```python
from build123d import *

# Parameters (mm, degrees)
F1_DEPTH = 8.382
F2_T     = 5.842
F3_W     = 7.7823624015
F3_H     = 6.8200882353
F3_W_2   = 7.1338275447
F3_H_2   = 5.8367699385
F3_W_3   = 11.938
F3_H_3   = 9.4247385517
F4_DEPTH = 5.842


with BuildPart() as f1:
    # F0 (on Front) → F1 (new body)
    with BuildSketch(Plane.XZ):
        with BuildLine():
            Line((-45.2634918147, -64.6201544654), (14.1725081853, -64.6201544654))
            ThreePointArc((14.1725081853, -64.6201544654), (18.6626362458, -62.760282526), (20.5225081853, -58.2701544654))
            Line((20.5225081853, -58.2701544654), (20.5225081853, 71.2698455346))
            ThreePointArc((20.5225081853, 71.2698455346), (18.6626362458, 75.7599735951), (14.1725081853, 77.6198455346))
            Line((14.1725081853, 77.6198455346), (-45.2634918147, 77.6198455346))
            ThreePointArc((-45.2634918147, 77.6198455346), (-49.7536198753, 75.7599735951), (-51.6134918147, 71.2698455346))
            Line((-51.6134918147, 71.2698455346), (-51.6134918147, -58.2701544654))
            ThreePointArc((-51.6134918147, -58.2701544654), (-49.7536198753, -62.760282526), (-45.2634918147, -64.6201544654))
        make_face()
    extrude(amount=F1_DEPTH)

    # F2
    f2_openings = [f1.faces().sort_by_distance(p)[0] for p in [
        (-15.545492, -8.382, 6.499846),
    ]]
    offset(amount=F2_T, openings=f2_openings, kind=Kind.INTERSECTION)

    # F3 (on face) → F4 (cut)
    with BuildSketch(Plane(origin=(0, 5.842, 0), x_dir=(-1, 0, 0), z_dir=(0, 1, 0))):
        with Locations((40.2088426054, 66.2087770264)):
            Rectangle(F3_W, F3_H)
        with Locations((3.5669137724, 66.7004361749)):
            Rectangle(F3_W_2, F3_H_2)
        with Locations((21.0826918147, 67.5111021847)):
            Rectangle(F3_W_3, F3_H_3)
    extrude(amount=-F4_DEPTH, mode=Mode.SUBTRACT)


solid = f1.part
```
Can you work these out from the model? Positions are in its coordinate system, mm. A direction names the side the tool comes from. Coordinates: 2 decimals unless noted, no trailing zeros. Write each loop counter-clockwise with the first axis right and the second up, starting at its lowest first coordinate (ties: lowest second). Pieces come first, ordered by that corner, then holes. Notation, with made-up numbers: (55, 76) - (70, 76) arc R28 cw to (70, 108) - close; hole circle Ø1 at (38, -15). An arc over 180 degrees is marked (long way). Return JSON: item names as keys, results as strings.
Q1. On a 3-axis mill with a long thin cutter (end or side, diameter ignored), from which of +Z, -Z, +X, -X, +Y, -Y can I reach the whole of each face in a straight line? I mean faces 1 (the cylindrical face through (-53.979, -1.17, -66.796)), 2 (the cylindrical face through (-49.704, -4.132, 75.809)), 3 (the flat face through (-15.114, 3, 67)). Say none if no direction works.
Computed values:
{"face 1": "-Z, -X, +Y, -Y", "face 2": "-Y", "face 3": "+Y, -Y"}
Q2. If we section it at C-C (x = 10): Please give me the cut outline in (y, z), then the cut area to 3 significant figures.
Computed values:
{"outline": "(-8.38, -70.46) - (5.84, -70.46) - (5.84, 83.46) - (-8.38, 83.46) - (-8.38, 77.62) - (0, 77.62) - (0, -64.62) - (-8.38, -64.62) - close", "area": "997 mm2"}
Q3. If we section it at B-B (y = 4.25): Please give me the cut outline in (x, z).
Computed values:
{"outline": "(-57.46, -58.27) arc R12.19 ccw to (-45.26, -70.46) - (14.17, -70.46) arc R12.19 ccw to (26.36, -58.27) - (26.36, 71.27) arc R12.19 ccw to (14.17, 83.46) - (-45.26, 83.46) arc R12.19 ccw to (-57.46, 71.27) - close; hole (-44.1, 62.8) - (-36.32, 62.8) - (-36.32, 69.62) - (-44.1, 69.62) - close; hole (-27.05, 62.8) - (-15.11, 62.8) - (-15.11, 72.22) - (-27.05, 72.22) - close; hole (-7.13, 63.78) - (0, 63.78) - (0, 69.62) - (-7.13, 69.62) - close"}
Q4. Thinking about a two-plate mould opening in Z: for faces 4 (the flat face through (-36.318, 3, 66)), 5 (the cylindrical face through (22.888, -1.17, 79.796)), 6 (the flat face through (-57.455, -1, 7)), which applies, +Z half, -Z half, draft (parallel to the pull), parting line (faces both ways), or undercut?
Computed values:
{"face 4": "undercut", "face 5": "+Z half", "face 6": "draft"}
Q5. If we section it at A-A (x = -5): Please give me the cut outline in (y, z), then the cut area to 3 significant figures.
Computed values:
{"outline": "(-8.38, -70.46) - (5.84, -70.46) - (5.84, 63.78) - (0, 63.78) - (0, -64.62) - (-8.38, -64.62) - close; (-8.38, 77.62) - (0, 77.62) - (0, 69.62) - (5.84, 69.62) - (5.84, 83.46) - (-8.38, 83.46) - close", "area": "963 mm2"}
Q6. If we section it at D-D (y = -2.75): Please give me the cut outline in (x, z), then the cut area to 3 significant figures.
Computed values:
{"outline": "(-57.46, -58.27) arc R12.19 ccw to (-45.26, -70.46) - (14.17, -70.46) arc R12.19 ccw to (26.36, -58.27) - (26.36, 71.27) arc R12.19 ccw to (14.17, 83.46) - (-45.26, 83.46) arc R12.19 ccw to (-57.46, 71.27) - close; hole (-51.61, -58.27) arc R6.35 ccw to (-45.26, -64.62) - (14.17, -64.62) arc R6.35 ccw to (20.52, -58.27) - (20.52, 71.27) arc R6.35 ccw to (14.17, 77.62) - (-45.26, 77.62) arc R6.35 ccw to (-51.61, 71.27) - close", "area": "2,550 mm2"}
Q7. I'm going to push a flat-ended pin straight in: pin 1 Ø21.5 at (x, z) = (-16.5, 22) entering from -Y. Where does the tip first touch, or does it pass through?
Computed values:
{"pin 1": "stops at y = 0"}
Q8. Please list where these lines run through material, in increasing order: L1, parallel to X at y = -4, z = 55.5; L2, parallel to Z at x = 12, y = -6; L3, parallel to Z at x = -2, y = 3.75. Write a range as from..to.
Computed values:
{"L1": "x = -57.46..-51.61, 20.52..26.36", "L2": "z = -70.46..-64.62, 77.62..83.46", "L3": "z = -70.46..63.78, 69.62..83.46"}
